```python
from build123d import *

# Parameters (mm, degrees)
SKETCH1_W           = 539
SKETCH1_H           = 299
BOSS_EXTRUDE1_DEPTH = 1.5
SKETCH10_W          = 70
SKETCH10_H          = 20
CUT_EXTRUDE6_DEPTH  = 309.192715683
SKETCH2_R           = 3
SKETCH2_R_2         = 2
CUT_EXTRUDE1_DEPTH  = 10
CUT_EXTRUDE3_DEPTH  = 309.192715683
CUT_EXTRUDE5_DEPTH  = 309.192715683
SKETCH7_W           = 15
SKETCH7_H           = 106.5
CUT_EXTRUDE4_DEPTH  = 309.192715683


with BuildPart() as part:
    # Sketch1 → Boss-Extrude1 (new body)
    with BuildSketch(Plane(origin=(0, 0, 0), x_dir=(1, 0, 0), z_dir=(0, 1, 0))):
        Rectangle(SKETCH1_W, SKETCH1_H)
    extrude(amount=-BOSS_EXTRUDE1_DEPTH)

    # Sketch10 → Cut-Extrude6 (cut, through all)
    with BuildSketch(Plane(origin=(0, 0, 0), x_dir=(1, 0, 0), z_dir=(0, 1, 0))):
        Polygon((269.5, 149.5), (199.5, 149.5), (199.5, 129.5), (249.5, 129.5), (249.5, 91.5), (269.5, 91.5), align=None)
        with Locations((234.5, -139.5)):
            Rectangle(SKETCH10_W, SKETCH10_H)
    extrude(amount=-CUT_EXTRUDE6_DEPTH, mode=Mode.SUBTRACT)

    # Sketch2 → Cut-Extrude1 (cut)
    with BuildSketch(Plane(origin=(0, 0, 0), x_dir=(1, 0, 0), z_dir=(0, 1, 0))):
        with Locations(Location((-260, 0, 0), (0, 0, 270))):
            Circle(SKETCH2_R)
        with Locations(Location((-260, 15, 0), (0, 0, 270))):
            Circle(SKETCH2_R_2)
        with Locations(Location((-260, -15, 0), (0, 0, 270))):
            Circle(SKETCH2_R_2)
    cut_extrude1 = extrude(amount=-CUT_EXTRUDE1_DEPTH, mode=Mode.SUBTRACT)

    # Mirror1: Cut-Extrude1 across plane
    add(cut_extrude1.mirror(Plane(origin=(0, 0, 0), x_dir=(0, 0, 1), z_dir=(1, 0, 0))), mode=Mode.SUBTRACT)

    # Sketch5 → Cut-Extrude3 (cut, through all)
    with BuildSketch(Plane(origin=(0, 0, 0), x_dir=(1, 0, 0), z_dir=(0, 1, 0))):
        Polygon((-100.5, -62.4), (-100.5, -84), (128.5, -84), (128.5, 84), (-100.5, 84), align=None)
    extrude(amount=-CUT_EXTRUDE3_DEPTH, mode=Mode.SUBTRACT)

    # Sketch9 → Cut-Extrude5 (cut, through all)
    with BuildSketch(Plane(origin=(0, 0, 0), x_dir=(1, 0, 0), z_dir=(0, 1, 0))):
        Polygon((-234.5, 3), (-228.5, 3), (-228.5, 83.5), (-130, 83.5), (-130, -99.5), (-95, -99.5), (-95, -134.5), (184.5, -134.5), (184.5, -114.5), (234.5, -114.5), (234.5, -3), (228.5, -3), (228.5, -108.5), (178.5, -108.5), (178.5, -128.5), (-89, -128.5), (-89, -93.5), (-110.5, -93.5), (-110.5, 89.5), (-234.5, 89.5), align=None)
    extrude(amount=-CUT_EXTRUDE5_DEPTH, mode=Mode.SUBTRACT)

    # Sketch7 → Cut-Extrude4 (cut, through all)
    with BuildSketch(Plane(origin=(0, 0, 0), x_dir=(1, 0, 0), z_dir=(0, 1, 0))):
        Polygon((-259.5, -13), (-218.5, -13), (-218.5, 73.5), (-140, 73.5), (-140, -109.5), (-105, -109.5), (-105, -139.5), (-140, -139.5), (-259.5, -139.5), align=None)
        Polygon((-259.5, 139.5), (-244.5, 139.5), (-100.5, 139.5), (189.5, 139.5), (189.5, 119.5), (239.5, 119.5), (239.5, 81.5), (259.5, 81.5), (259.5, 13), (218.5, 13), (218.5, -101.728673951), (169.107799643, -101.728673951), (169.107799643, -118.5), (-79, -118.5), (-79, -94), (138.5, -94), (138.5, 94), (-100.5, 94), (-100.5, 99.5), (-244.5, 99.5), (-244.5, 13), (-259.5, 13), align=None)
        with Locations((252, -66.25)):
            Rectangle(SKETCH7_W, SKETCH7_H)
    extrude(amount=-CUT_EXTRUDE4_DEPTH, mode=Mode.SUBTRACT)


solid = part.part
```
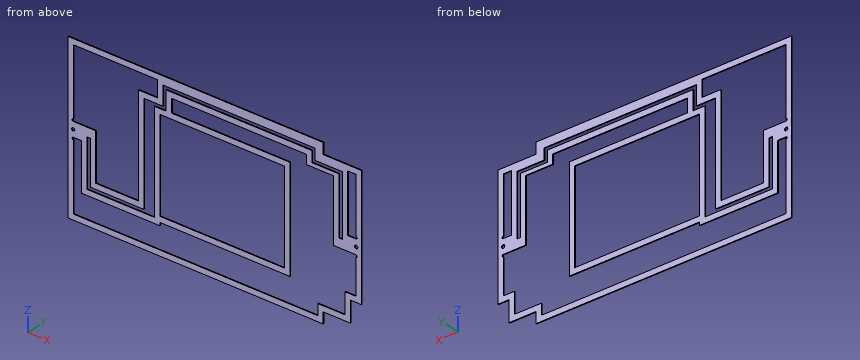
Geometry check sheet. Reference: the model listing, model coordinates, mm. Coordinates: 2 decimals unless noted, no trailing zeros. Order: outer loops, then holes, each group sorted by start corner. A loop starts at its lowest first (then second) coordinate and runs counter-clockwise, first axis right, second up.
Q1. Depth check by flat-ended pin: pin 1 Ø0.8 at (x, y) = (216, -0.5) entering from -Z; pin 2 Ø3.5 at (x, z) = (260, -15) entering from +Y; pin 3 Ø0.8 at (x, y) = (254, -0.5) entering from +Z. Enter the tip coordinate at first touch or a pass-through.
Reply:
pin 1: stops at z = -129.5
pin 2: passes through
pin 3: stops at z = 129.5
Q2. Sectioned sample at A-A on z = 72. Record the cut outline in (x, y), and give its area (3 significant figures).
Reply:
outline: (-269.5, -1.5) - (-259.5, -1.5) - (-259.5, 0) - (-269.5, 0) - close; (-140, -1.5) - (-130, -1.5) - (-130, 0) - (-140, 0) - close; (-110.5, -1.5) - (-100.5, -1.5) - (-100.5, 0) - (-110.5, 0) - close; (128.5, -1.5) - (138.5, -1.5) - (138.5, 0) - (128.5, 0) - close; (218.5, -1.5) - (228.5, -1.5) - (228.5, 0) - (218.5, 0) - close; (234.5, -1.5) - (244.5, -1.5) - (244.5, 0) - (234.5, 0) - close; (259.5, -1.5) - (269.5, -1.5) - (269.5, 0) - (259.5, 0) - close
area: 105 mm2
Q3. Thickness scan on probe 1 along Z at (x, y) = (260, -1.2); probe 2 along Z at (x, y) = (-260, -0.55); probe 3 along X at (y, z) = (-1.4, 102). Record the ranges inside material, lowest first.
Reply:
probe 1: z = -91.5 to -17, -13 to -3, 3 to 13, 17 to 129.5
probe 2: z = -149.5 to -17, -13 to -3, 3 to 13, 17 to 149.5
probe 3: x = -269.5 to -259.5, -140 to -95, -89 to -79, 169.11 to 228.5, 234.5 to 244.5, 259.5 to 269.5
Q4. Sectioned sample at B-B on x = -158. Record the cut outline in (y, z).
Reply:
outline: (-1.5, -149.5) - (0, -149.5) - (0, -139.5) - (-1.5, -139.5) - close; (-1.5, -99.5) - (0, -99.5) - (0, -89.5) - (-1.5, -89.5) - close; (-1.5, -83.5) - (0, -83.5) - (0, -73.5) - (-1.5, -73.5) - close; (-1.5, 139.5) - (0, 139.5) - (0, 149.5) - (-1.5, 149.5) - close
Q5. Sectioned sample at C-C on y = -0.4. Give the number of separate pieces and of enclosed holes in the cut face, and give its area (3 significant figures).
Reply:
separate pieces: 1
enclosed holes: 7
area: 40,000 mm2
